from build123d import *

# Parameters (mm, degrees)
ESQUISSE1_W                                  = 50
ESQUISSE1_H                                  = 64
BOSS_EXTRU_1_DEPTH                           = 30
ESQUISSE2_W                                  = 58.443807101
ESQUISSE2_H                                  = 34.604437798
ENL_V_MAT_EXTRU_1_DEPTH                      = 75.973328591
D_GAGEMENT_M41_D                             = 4.5
D_GAGEMENT_M42_D                             = 4.5
CHAMBRAGE_POUR_VIS_T_TE_RONDE_BOMB_2_COUNT   = 2
CHAMBRAGE_POUR_VIS_T_TE_RONDE_BOMB_2_PITCH   = 20.75901561
CHAMBRAGE_POUR_VIS_T_TE_RONDE_BOMB_3_COUNT   = 2
CHAMBRAGE_POUR_VIS_T_TE_RONDE_BOMB_3_PITCH   = 18.074069798
CHAMBRAGE_POUR_VIS_T_TE_RONDE_BOMB_4_COUNT   = 2
CHAMBRAGE_POUR_VIS_T_TE_RONDE_BOMB_4_PITCH   = 27.524693062
CHAMBRAGE_POUR_VIS_T_TE_RONDE_BOMB_5_COUNT   = 2
CHAMBRAGE_POUR_VIS_T_TE_RONDE_BOMB_5_PITCH   = 39.238665714
CHAMBRAGE_POUR_VIS_T_TE_RONDE_BOMB_6_COUNT   = 2
CHAMBRAGE_POUR_VIS_T_TE_RONDE_BOMB_6_PITCH   = 44.391548927
CHAMBRAGE_POUR_VIS_T_TE_RONDE_BOMB_7_A_COUNT = 2
CHAMBRAGE_POUR_VIS_T_TE_RONDE_BOMB_7_A_PITCH = 20


with BuildPart() as part:
    # Esquisse1 → Boss.-Extru.1 (new body)
    with BuildSketch(Plane.XY):
        Rectangle(ESQUISSE1_W, ESQUISSE1_H)
    extrude(amount=BOSS_EXTRU_1_DEPTH)

    # Esquisse2 → Enlèv. mat.-Extru.1 (cut, through all)
    with BuildSketch(Plane(origin=(0, 32, 0), x_dir=(1, 0, 0), z_dir=(0, 1, 0))):
        with Locations((9.221903551, -22.302218899)):
            Rectangle(ESQUISSE2_W, ESQUISSE2_H)
    extrude(amount=-ENL_V_MAT_EXTRU_1_DEPTH, mode=Mode.SUBTRACT)

    # Dégagement M41 (through all)
    with Locations(Plane(origin=(0, 0, 0), x_dir=(-1, 0, 0), z_dir=(0, 0, -1))):
        with Locations((6.838730229, 18.937151978), (-13.92028538, 18.937151978), (-13.92028538, 0.86308218), (6.838730229, 0.86308218), (6.838730229, -20.301513736), (-13.92028538, -20.301513736)):
            Hole(D_GAGEMENT_M41_D / 2)

    # Dégagement M42 (through all)
    with Locations(Plane.ZY.offset(25)):
        with Locations((20, 14.5), (20, -5.5)):
            Hole(D_GAGEMENT_M42_D / 2)

    # Esquisse7 → Chambrage pour vis _ t_te ronde bomb_e M (revolve, cut)
    with BuildSketch(Plane(origin=(13.92028538, 18.937151978, 5), x_dir=(0, -1, 0), z_dir=(1, 0, 0))):
        Polygon((0, 0), (0, 5), (2.25, 5), (2.25, 3.125), (2.275, 3.1), (4.5, 3.1), (4.5, 0), align=None)
    chambrage_pour_vis_t_te_ronde_bomb_e_m = revolve(axis=Axis((13.92028538, 18.937151978, 11.35), (0, 0, -1)), mode=Mode.SUBTRACT)

    # Chambrage pour vis _ t_te ronde bomb 2: Chambrage pour vis _ t_te ronde bomb_e M ×2
    with Locations(*[(-i * CHAMBRAGE_POUR_VIS_T_TE_RONDE_BOMB_2_PITCH, 0, 0) for i in range(1, CHAMBRAGE_POUR_VIS_T_TE_RONDE_BOMB_2_COUNT)]):
        add(chambrage_pour_vis_t_te_ronde_bomb_e_m, mode=Mode.SUBTRACT)

    # Chambrage pour vis _ t_te ronde bomb 3: Chambrage pour vis _ t_te ronde bomb_e M ×2
    with Locations(*[(0, -i * CHAMBRAGE_POUR_VIS_T_TE_RONDE_BOMB_3_PITCH, 0) for i in range(1, CHAMBRAGE_POUR_VIS_T_TE_RONDE_BOMB_3_COUNT)]):
        add(chambrage_pour_vis_t_te_ronde_bomb_e_m, mode=Mode.SUBTRACT)

    # Chambrage pour vis _ t_te ronde bomb 4: Chambrage pour vis _ t_te ronde bomb_e M ×2
    with Locations(*[Vector(-0.7541960799735443, -0.6566492769755702, 0) * (i * CHAMBRAGE_POUR_VIS_T_TE_RONDE_BOMB_4_PITCH) for i in range(1, CHAMBRAGE_POUR_VIS_T_TE_RONDE_BOMB_4_COUNT)]):
        add(chambrage_pour_vis_t_te_ronde_bomb_e_m, mode=Mode.SUBTRACT)

    # Chambrage pour vis _ t_te ronde bomb 5: Chambrage pour vis _ t_te ronde bomb_e M ×2
    with Locations(*[(0, -i * CHAMBRAGE_POUR_VIS_T_TE_RONDE_BOMB_5_PITCH, 0) for i in range(1, CHAMBRAGE_POUR_VIS_T_TE_RONDE_BOMB_5_COUNT)]):
        add(chambrage_pour_vis_t_te_ronde_bomb_e_m, mode=Mode.SUBTRACT)

    # Chambrage pour vis _ t_te ronde bomb 6: Chambrage pour vis _ t_te ronde bomb_e M ×2
    with Locations(*[Vector(-0.46763440590484284, -0.8839219775602509, 0) * (i * CHAMBRAGE_POUR_VIS_T_TE_RONDE_BOMB_6_PITCH) for i in range(1, CHAMBRAGE_POUR_VIS_T_TE_RONDE_BOMB_6_COUNT)]):
        add(chambrage_pour_vis_t_te_ronde_bomb_e_m, mode=Mode.SUBTRACT)

    # Esquisse9 → Chambrage pour vis _ t_te ronde bomb 7 (revolve, cut)
    with BuildSketch(Plane(origin=(-20, 14.5, 20), x_dir=(0, 0, -1), z_dir=(0, 1, 0))):
        Polygon((0, 0), (0, 5), (2.25, 5), (2.25, 3.125), (2.275, 3.1), (4.5, 3.1), (4.5, 0), align=None)
    chambrage_pour_vis_t_te_ronde_bomb_7 = revolve(axis=Axis((-13.65, 14.5, 20), (-1, 0, 0)), mode=Mode.SUBTRACT)

    # Chambrage pour vis _ t_te ronde bomb 7 a: Chambrage pour vis _ t_te ronde bomb 7 ×2
    with Locations(*[(0, -i * CHAMBRAGE_POUR_VIS_T_TE_RONDE_BOMB_7_A_PITCH, 0) for i in range(1, CHAMBRAGE_POUR_VIS_T_TE_RONDE_BOMB_7_A_COUNT)]):
        add(chambrage_pour_vis_t_te_ronde_bomb_7, mode=Mode.SUBTRACT)


solid = part.part
Model file for the job. Use its own axes, mm. A direction names the side the tool comes from. Give positions to 0.01 mm unless a question says otherwise; leave off trailing zeros. Order: outer loops, then holes, each group sorted by start corner. A loop starts at its lowest first (then second) coordinate and runs counter-clockwise, first axis right, second up. Notation, with made-up numbers: (-24.5, 75) - (16.5, 75) arc R22 ccw to (16.5, 102) - close; hole circle Ø2 at (50.5, 11). An arc over 180 degrees is marked (long way). Return JSON: item names as keys, results as strings.
1) Cut at C-C, the plane y = -13.5. Give the cut face in (x, z).
Geometry says:
{"outline": "(-25, 0) - (25, 0) - (25, 5) - (-20, 5) - (-20, 30) - (-25, 30) - close"}
2) Flat gauge pins, fed straight in: P1, Ø4.5, axis at x = -5, y = -1, coming from the +Z side; P2, Ø6, axis at x = -6.84, y = 18.94, coming from the +Z side; P3, Ø1, axis at y = 15.5, z = 6, coming from the +X side. Where does each tip first touch, or does it go through?
Geometry says:
{"P1": "z = 5", "P2": "z = 1.9", "P3": "x = -20"}
3) Probe line 1 (Z direction, x = -24.4, y = -5.5); line 2 (Z direction, x = 19, y = -20); line 3 (X direction, y = 9, z = 16.25). List the from-to ranges inside material, lowest first. Write a range as from..to.
Geometry says:
{"line 1": "0..17.75, 22.25..30", "line 2": "0..5", "line 3": "-25..-20"}
4) 3-axis set-ups, long thin cutter, end or side, ignore diameter. For faces 1 (the cylindrical face through (-21.53, 11.46, 23.32)), 2 (the flat face through (16, -18, 1.9)), 3 (the flat face through (-20, 0, 18)): which of +Z, -Z, +X, -X, +Y, -Y reach the whole face in a straight line?
Geometry says:
{"face 1": "+X", "face 2": "+Z", "face 3": "+Z, +X, +Y, -Y"}
5) Cut at D-D, the plane x = 12.5. Count the separate pieces of the cut face and the enclosed holes in it, plus the area to 3 significant figures.
Geometry says:
{"separate pieces": "4", "enclosed holes": "0", "area": "221 mm²"}
6) Pull direction Z, two halves, no side cores. Call faces 4 (the flat face through (-23.1, -8, 19)), 5 (the flat face through (-5, 3, 1.9)), 6 (the cylindrical face through (9.46, -19.72, 3.47)): pulls with the +Z half, pulls with the -Z half, needs draft (parallel to the pull), parting line crosses it, or undercut.
Geometry says:
{"face 4": "undercut", "face 5": "pulls with the +Z half", "face 6": "needs draft"}
7) Cut at A-A, the plane z = 20. Give the cut face in (x, y) (3 decimals), plus the area to 3 significant figures.
Geometry says:
{"outline": "(-25, -32) - (-20, -32) - (-20, -10) - (-23.1, -10) - (-23.1, -7.775) - (-23.125, -7.75) - (-25, -7.75) - close; (-25, -3.25) - (-23.125, -3.25) - (-23.1, -3.225) - (-23.1, -1) - (-20, -1) - (-20, 10) - (-23.1, 10) - (-23.1, 12.225) - (-23.125, 12.25) - (-25, 12.25) - close; (-25, 16.75) - (-23.125, 16.75) - (-23.1, 16.775) - (-23.1, 19) - (-20, 19) - (-20, 32) - (-25, 32) - close", "area": "247 mm²"}
8) Cut at B-B, the plane y = -5.5. Give the cut face in (x, z) (3 decimals).
Geometry says:
{"outline": "(-25, 0) - (25, 0) - (25, 5) - (-20, 5) - (-20, 15.5) - (-23.1, 15.5) - (-23.1, 17.725) - (-23.125, 17.75) - (-25, 17.75) - close; (-25, 22.25) - (-23.125, 22.25) - (-23.1, 22.275) - (-23.1, 24.5) - (-20, 24.5) - (-20, 30) - (-25, 30) - close"}
